```python
from build123d import *

# Parameters (mm, degrees)
SKETCH1_W           = 28
SKETCH1_H           = 28
BOSS_EXTRUDE1_DEPTH = 25
SKETCH2_W           = 28
SKETCH2_H           = 22
CUT_EXTRUDE1_DEPTH  = 22
SKETCH3_W           = 6.8
SKETCH3_H           = 22
CUT_EXTRUDE2_DEPTH  = 46.299006612
SKETCH4_R           = 2.35
CUT_EXTRUDE3_DEPTH  = 44.508619836
SKETCH5_W           = 28
SKETCH5_H           = 6
CUT_EXTRUDE4_DEPTH  = 4


with BuildPart() as part:
    # Sketch1 → Boss-Extrude1 (new body)
    with BuildSketch(Plane(origin=(0, 0, 0), x_dir=(1, 0, 0), z_dir=(0, 1, 0))):
        with Locations((14, -14)):
            Rectangle(SKETCH1_W, SKETCH1_H)
    extrude(amount=BOSS_EXTRUDE1_DEPTH)

    # Sketch2 → Cut-Extrude1 (cut)
    with BuildSketch(Plane(origin=(0, 25, 0), x_dir=(1, 0, 0), z_dir=(0, 1, 0))):
        with Locations((14, -11)):
            Rectangle(SKETCH2_W, SKETCH2_H)
    extrude(amount=-CUT_EXTRUDE1_DEPTH, mode=Mode.SUBTRACT)

    # Sketch3 → Cut-Extrude2 (cut, through all)
    with BuildSketch(Plane(origin=(0, 3, 0), x_dir=(1, 0, 0), z_dir=(0, 1, 0))):
        with Locations((14, -11)):
            Rectangle(SKETCH3_W, SKETCH3_H)
    extrude(amount=-CUT_EXTRUDE2_DEPTH, mode=Mode.SUBTRACT)

    # Sketch4 → Cut-Extrude3 (cut, through all)
    with BuildSketch(Plane(origin=(0, 0, 22), x_dir=(-1, 0, 0), z_dir=(0, 0, -1))):
        with Locations((-14, 10)):
            Circle(SKETCH4_R)
    extrude(amount=-CUT_EXTRUDE3_DEPTH, mode=Mode.SUBTRACT)

    # Sketch5 → Cut-Extrude4 (cut)
    with BuildSketch(Plane(origin=(0, 25, 0), x_dir=(1, 0, 0), z_dir=(0, 1, 0))):
        with Locations((14, -25)):
            Rectangle(SKETCH5_W, SKETCH5_H)
    extrude(amount=-CUT_EXTRUDE4_DEPTH, mode=Mode.SUBTRACT)


solid = part.part
```
Geometry: final body of the model. Coordinates: model frame, mm. A direction names the side the tool comes from. Give positions to 0.01 mm unless a question says otherwise; leave off trailing zeros. Loops run counter-clockwise (first coordinate to the right, second up) from the corner with the lowest first, then second, coordinate; pieces in that order, holes last. Notation, with made-up numbers: (9.25, 18.25) -> (33.25, 18.25) arc R19 ccw to (33.25, 33.25) -> close; hole circle Ø6 at (55, 66.25). An arc over 180 degrees is marked (long way). Return JSON: item names as keys, results as strings.
Item 1: Section A-A, the plane x = 14. Output: boundary loops of the cut face in (y, z).
Filled in:
{"outline": "(0, 22) -> (7.65, 22) -> (7.65, 28) -> (0, 28) -> close; (12.35, 22) -> (21, 22) -> (21, 28) -> (12.35, 28) -> close"}
Item 2: Section C-C, the plane z = 24.75. Output: boundary loops of the cut face in (x, y), plus the area to 3 significant figures.
Filled in:
{"outline": "(0, 0) -> (28, 0) -> (28, 21) -> (0, 21) -> close; hole circle Ø4.7 at (14, 10)", "area": "571 mm^2"}
Item 3: Section D-D, the plane x = 10. Output: boundary loops of the cut face in (y, z), plus the area to 3 significant figures.
Filled in:
{"outline": "(0, 0) -> (3, 0) -> (3, 22) -> (21, 22) -> (21, 28) -> (0, 28) -> close", "area": "192 mm^2"}
Item 4: Line query: line 1 (Y direction, x = 14, z = 24.9); line 2 (Y direction, x = 8.25, z = 11.5); line 3 (Z direction, x = 11.5, y = 19.5). Output: solid intervals per line, ascending.
Filled in:
{"line 1": "0 to 7.65, 12.35 to 21", "line 2": "0 to 3", "line 3": "22 to 28"}
Item 5: Section B-B, the plane y = 10. Output: boundary loops of the cut face in (x, z).
Filled in:
{"outline": "(0, 22) -> (11.65, 22) -> (11.65, 28) -> (0, 28) -> close; (16.35, 22) -> (28, 22) -> (28, 28) -> (16.35, 28) -> close"}
Item 6: Pin query (flat end, axial travel): P1, Ø3, axis at x = 23.5, z = 12.5, coming from the +Y side; P2, Ø10.5, axis at x = 10.5, y = 13.5, coming from the -Z side; P3, Ø4, axis at x = 14, y = 10, coming from the +Z side. Return the tip coordinate at first contact, or that it passes through.
Filled in:
{"P1": "y = 3", "P2": "z = 22", "P3": "through"}
Item 7: Access query for faces 5 (the flat face through (5, 3, 11)), 6 (the flat face through (28, 8.1, 22.4)), 7 (the flat face through (10.6, 2, 11)). Directions: +Z, -Z, +X, -X, +Y, -Y. A direction counts if a zero-diameter tool reaches every point of the face in a straight line with its end or side. Return the directions, or none.
Filled in:
{"face 5": "-Z, +X, -X, +Y", "face 6": "+Z, -Z, +X, +Y, -Y", "face 7": "-Z, +Y, -Y"}
Item 8: Mould query, pull axis X, two halves, no side actions, for faces 1 (the flat face through (0, 8.1, 22.4)), 2 (the flat face through (5, 1, 0)), 3 (the cylindrical face through (15.865, 8.57, 24.958)), 4 (the flat face through (17.4, 2, 11)). Classes: released by +X, released by -X, zero draft, split by the parting line, or undercut.
Filled in:
{"face 1": "released by -X", "face 2": "zero draft", "face 3": "undercut", "face 4": "undercut"}
